Work out the finished part from the listing and answer in its coordinate system (mm). Coordinates: 2 decimals unless noted, no trailing zeros. Write each loop counter-clockwise with the first axis right and the second up, starting at its lowest first coordinate (ties: lowest second). Pieces come first, ordered by that corner, then holes. Notation, with made-up numbers: (3, -33.75) - (40, -33.75) arc R32 ccw to (40, -6.75) - close; hole circle Ø3 at (-31.5, 0). An arc over 180 degrees is marked (long way). Use a Markdown table: item, result. Add a question column.
(1) The part is cut by section B-B, the plane z = 30. Give the vertices of the cut face in (x, y).
(2) The part is cut by section D-D, the plane z = -25. Give the vertices of the cut face in (x, y).
(3) The part is cut by section A-A, the plane x = 0. State how many separate pieces and enclosed holes the cut face has, then the cut area to 3 significant figures.
(4) The part is cut by section C-C, the plane z = 0. Give the vertices of the cut face in (x, y).
(5) Find the intervals of material crossed by line 1 (Z direction, x = 34.5, y = 3.05); line 2 (X direction, y = 3.35, z = 33); line 3 (X direction, y = 3, z = -15), in increasing order. Write a range as from..to.
(6) Given pin 1 Ø2.5 at (x, z) = (0, -30) entering from -Y; pin 2 Ø1 at (y, z) = (1, -10.5) entering from +X, each flat-ended and moving along its own axis, determine where each tip first touches the part or whether it passes through.
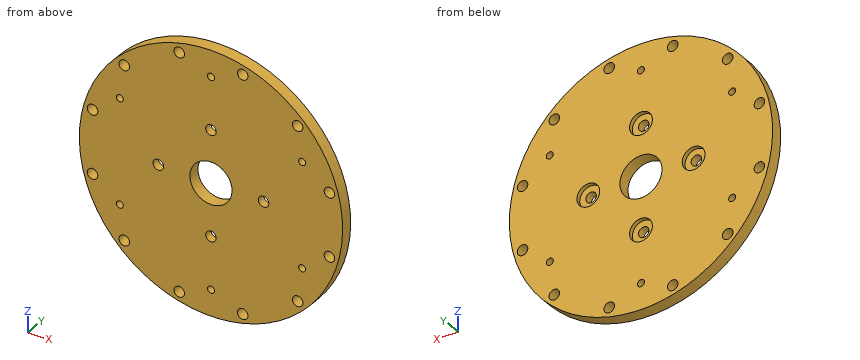
from build123d import *

# Parameters (mm, degrees)
SKETCH1_R           = 37.5
SKETCH1_R_2         = 6
SKETCH1_R_3         = 1.5
SKETCH1_R_4         = 1
BOSS_EXTRUDE1_DEPTH = 3.5
SKETCH2_R           = 3.25
CUT_EXTRUDE1_DEPTH  = 1.2


with BuildPart() as part:
    # Sketch1 → Boss-Extrude1 (new body)
    with BuildSketch(Plane(origin=(0, 0, 0), x_dir=(1, 0, 0), z_dir=(0, 1, 0))):
        with Locations(Location((0, 0, 0), (0, 0, 270))):
            Circle(SKETCH1_R)
        with Locations(Location((0, 0, 0), (0, 0, 270))):
            Circle(SKETCH1_R_2, mode=Mode.SUBTRACT)
        with Locations(Location((0, 15, 0), (0, 0, 270))):
            Circle(SKETCH1_R_3, mode=Mode.SUBTRACT)
        with Locations(Location((15, 0, 0), (0, 0, 270))):
            Circle(SKETCH1_R_3, mode=Mode.SUBTRACT)
        with Locations(Location((0, -15, 0), (0, 0, 270))):
            Circle(SKETCH1_R_3, mode=Mode.SUBTRACT)
        with Locations(Location((-15, 0, 0), (0, 0, 270))):
            Circle(SKETCH1_R_3, mode=Mode.SUBTRACT)
        with Locations(Location((-33.737040436, -9.03981274, 0), (0, 0, 270))):
            Circle(SKETCH1_R_3, mode=Mode.SUBTRACT)
        with Locations(Location((-33.737040436, 9.03981274, 0), (0, 0, 270))):
            Circle(SKETCH1_R_3, mode=Mode.SUBTRACT)
        with Locations(Location((-24.697227696, 24.697227696, 0), (0, 0, 270))):
            Circle(SKETCH1_R_3, mode=Mode.SUBTRACT)
        with Locations(Location((-9.03981274, 33.737040436, 0), (0, 0, 270))):
            Circle(SKETCH1_R_3, mode=Mode.SUBTRACT)
        with Locations(Location((9.03981274, 33.737040436, 0), (0, 0, 270))):
            Circle(SKETCH1_R_3, mode=Mode.SUBTRACT)
        with Locations(Location((24.697227696, 24.697227696, 0), (0, 0, 270))):
            Circle(SKETCH1_R_3, mode=Mode.SUBTRACT)
        with Locations(Location((33.737040436, 9.03981274, 0), (0, 0, 270))):
            Circle(SKETCH1_R_3, mode=Mode.SUBTRACT)
        with Locations(Location((33.737040436, -9.03981274, 0), (0, 0, 270))):
            Circle(SKETCH1_R_3, mode=Mode.SUBTRACT)
        with Locations(Location((24.697227696, -24.697227696, 0), (0, 0, 270))):
            Circle(SKETCH1_R_3, mode=Mode.SUBTRACT)
        with Locations(Location((9.03981274, -33.737040436, 0), (0, 0, 270))):
            Circle(SKETCH1_R_3, mode=Mode.SUBTRACT)
        with Locations(Location((-9.03981274, -33.737040436, 0), (0, 0, 270))):
            Circle(SKETCH1_R_3, mode=Mode.SUBTRACT)
        with Locations(Location((-24.697227696, -24.697227696, 0), (0, 0, 270))):
            Circle(SKETCH1_R_3, mode=Mode.SUBTRACT)
        with Locations(Location((0, 30, 0), (0, 0, 270))):
            Circle(SKETCH1_R_4, mode=Mode.SUBTRACT)
        with Locations(Location((25.980762114, 15, 0), (0, 0, 270))):
            Circle(SKETCH1_R_4, mode=Mode.SUBTRACT)
        with Locations(Location((25.980762114, -15, 0), (0, 0, 270))):
            Circle(SKETCH1_R_4, mode=Mode.SUBTRACT)
        with Locations(Location((0, -30, 0), (0, 0, 270))):
            Circle(SKETCH1_R_4, mode=Mode.SUBTRACT)
        with Locations(Location((-25.980762114, -15, 0), (0, 0, 270))):
            Circle(SKETCH1_R_4, mode=Mode.SUBTRACT)
        with Locations(Location((-25.980762114, 15, 0), (0, 0, 270))):
            Circle(SKETCH1_R_4, mode=Mode.SUBTRACT)
    extrude(amount=BOSS_EXTRUDE1_DEPTH)

    # Sketch2 → Cut-Extrude1 (cut)
    with BuildSketch(Plane(origin=(0, 3.5, 0), x_dir=(1, 0, 0), z_dir=(0, 1, 0))):
        with Locations(Location((0, 15, 0), (0, 0, 270))):
            Circle(SKETCH2_R)
        with Locations(Location((15, 0, 0), (0, 0, 270))):
            Circle(SKETCH2_R)
        with Locations(Location((0, -15, 0), (0, 0, 270))):
            Circle(SKETCH2_R)
        with Locations(Location((-15, 0, 0), (0, 0, 270))):
            Circle(SKETCH2_R)
    extrude(amount=-CUT_EXTRUDE1_DEPTH, mode=Mode.SUBTRACT)


solid = part.part
Model answer:
| question | item | result |
|---|---|---|
| 1 | outline | (-22.5, 0) - (-1, 0) - (-1, 3.5) - (-22.5, 3.5) - close; (1, 0) - (22.5, 0) - (22.5, 3.5) - (1, 3.5) - close |
| 2 | outline | (-27.95, 0) - (-26.17, 0) - (-26.17, 3.5) - (-27.95, 3.5) - close; (-23.23, 0) - (23.23, 0) - (23.23, 3.5) - (-23.23, 3.5) - close; (26.17, 0) - (27.95, 0) - (27.95, 3.5) - (26.17, 3.5) - close |
| 3 | separate pieces | 6 |
| 3 | enclosed holes | 0 |
| 3 | area | 177 mm^2 |
| 4 | outline | (-37.5, 0) - (-16.5, 0) - (-16.5, 2.3) - (-18.25, 2.3) - (-18.25, 3.5) - (-37.5, 3.5) - close; (-13.5, 0) - (-6, 0) - (-6, 3.5) - (-11.75, 3.5) - (-11.75, 2.3) - (-13.5, 2.3) - close; (6, 0) - (13.5, 0) - (13.5, 2.3) - (11.75, 2.3) - (11.75, 3.5) - (6, 3.5) - close; (16.5, 0) - (37.5, 0) - (37.5, 3.5) - (18.25, 3.5) - (18.25, 2.3) - (16.5, 2.3) - close |
| 5 | line 1 | -14.7..-10.33, -7.75..7.75, 10.33..14.7 |
| 5 | line 2 | -17.81..-10.35, -7.73..7.73, 10.35..17.81 |
| 5 | line 3 | -34.37..-26.98, -24.98..-3.25, 3.25..24.98, 26.98..34.37 |
| 6 | pin 1 | y = 0 |
| 6 | pin 2 | x = 36.14 |
